```python
from build123d import *

# Parameters (mm, degrees)
SKETCH493_R     = 0.875
PAD402_DEPTH    = 1
POCKET036_DEPTH = 1.3
PAD_DEPTH       = 0.9
POCKET_DEPTH    = 2.5
CHAMFER_SIZE    = 0.1


with BuildPart() as part:
    # Sketch493 → Pad402 (new body, symmetric)
    with BuildSketch(Plane(origin=(50, -50, 0.5), x_dir=(1, 0, 0), z_dir=(0, 0, 1))):
        with BuildLine():
            Line((-53.3, 47.9), (-53.3, 46.1))
            Line((-53.3, 46.1), (-52.917836, 46.1))
            ThreePointArc((-52.73607, 46.021642), (-52.818868, 46.079576), (-52.917836, 46.1))
            ThreePointArc((-52.73607, 46.021642), (-52.488396, 45.812963), (-52.2, 45.665599))
            Line((-52.2, 45.665599), (-52.2, 45.141069))
            ThreePointArc((-52.2, 45.141069), (-50.38471, 45.594427), (-49.812013, 47.375671))
            ThreePointArc((-47.375671, 49.812013), (-49.245018, 49.245018), (-49.812013, 47.375671))
            ThreePointArc((-47.375671, 49.812013), (-45.594427, 50.38471), (-45.141069, 52.2))
            Line((-45.665599, 52.2), (-45.141069, 52.2))
            ThreePointArc((-45.665599, 52.2), (-45.812963, 52.488396), (-46.021642, 52.73607))
            ThreePointArc((-46.1, 52.917836), (-46.079576, 52.818868), (-46.021642, 52.73607))
            Line((-46.1, 53.3), (-46.1, 52.917836))
            Line((-47.9, 53.3), (-46.1, 53.3))
            Line((-47.9, 53.3), (-47.9, 52.917836))
            ThreePointArc((-47.978358, 52.73607), (-47.920424, 52.818868), (-47.9, 52.917836))
            ThreePointArc((-47.978358, 52.73607), (-48.187037, 52.488396), (-48.334401, 52.2))
            Line((-48.334401, 52.2), (-51.75, 52.2))
            ThreePointArc((-51.75, 52.2), (-52.068198, 52.068198), (-52.2, 51.75))
            Line((-52.2, 51.75), (-52.2, 48.334401))
            ThreePointArc((-52.2, 48.334401), (-52.488396, 48.187037), (-52.73607, 47.978358))
            ThreePointArc((-52.917836, 47.9), (-52.818868, 47.920424), (-52.73607, 47.978358))
            Line((-52.917836, 47.9), (-53.3, 47.9))
        make_face()
        with Locations((-50, 50)):
            Circle(SKETCH493_R, mode=Mode.SUBTRACT)
    extrude(amount=PAD402_DEPTH, both=True)

    # Sketch494 → Pocket036 (cut)
    with BuildSketch(Plane(origin=(50, -50, 1.5), x_dir=(1, 0, 0), z_dir=(0, 0, 1))):
        with BuildLine():
            Line((0, 0), (-100, 0))
            Line((-100, 0), (-100, 51.8))
            ThreePointArc((-51.8, 100), (-85.882547, 85.882547), (-100, 51.8))
            Line((-51.8, 100), (0, 100))
            Line((0, 100), (0, 0))
        make_face()
    extrude(amount=-POCKET036_DEPTH, mode=Mode.SUBTRACT)

    # Sketch497 → Pad (join)
    with BuildSketch(Plane(origin=(50, -50, 0), x_dir=(1, 0, 0), z_dir=(0, 0, 1))):
        with BuildLine():
            Line((-53.3, 47.9), (-53.3, 46.1))
            Line((-53.3, 46.1), (-52.917836, 46.1))
            ThreePointArc((-52.73607, 46.021642), (-52.818868, 46.079576), (-52.917836, 46.1))
            ThreePointArc((-52.73607, 46.021642), (-50.275, 47), (-52.73607, 47.978358))
            ThreePointArc((-52.917836, 47.9), (-52.818868, 47.920424), (-52.73607, 47.978358))
            Line((-52.917836, 47.9), (-53.3, 47.9))
        make_face()
        with BuildLine():
            Line((-46.1, 53.3), (-46.1, 52.917836))
            ThreePointArc((-46.1, 52.917836), (-46.079576, 52.818868), (-46.021642, 52.73607))
            ThreePointArc((-47.978358, 52.73607), (-47, 50.275), (-46.021642, 52.73607))
            ThreePointArc((-47.978358, 52.73607), (-47.920424, 52.818868), (-47.9, 52.917836))
            Line((-47.9, 53.3), (-47.9, 52.917836))
            Line((-47.9, 53.3), (-46.1, 53.3))
        make_face()
    extrude(amount=-PAD_DEPTH)

    # Sketch → Pocket (cut, symmetric)
    with BuildSketch(Plane(origin=(50, -50, 0), x_dir=(1, 0, 0), z_dir=(0, 0, 1))):
        Polygon((-52.2, 44.2), (-44.2, 52.2), (-42, 52.2), (-52.2, 42), align=None)
    extrude(amount=POCKET_DEPTH, both=True, mode=Mode.SUBTRACT)

    # Chamfer
    chamfer_edges = [part.edges().sort_by_distance(p)[0] for p in [
        (4.15, 0.55, 0.2),
        (4.878226, 1.278226, -0.15),
        (4.15, 0.55, -0.5),
        (3.421774, -0.178226, -0.15),
        (-0.55, -4.15, 0.2),
        (0.178226, -3.421774, -0.15),
        (-0.55, -4.15, -0.5),
        (-1.278226, -4.878226, -0.15),
    ]]
    chamfer(chamfer_edges, length=CHAMFER_SIZE)


solid = part.part
```
Model file for the job. Use its own axes, mm. A direction names the side the tool comes from. Give positions to 0.01 mm unless a question says otherwise; leave off trailing zeros. Order: outer loops, then holes, each group sorted by start corner. A loop starts at its lowest first (then second) coordinate and runs counter-clockwise, first axis right, second up.
1) Saw through at C-C, the plane y = -0.75. Write the cut outline in (x, z), then the cut area to 3 significant figures.
2) Saw through at D-D, the plane x = 3. Write the cut outline in (y, z) (3 decimals), then the cut area to 3 significant figures.
3) Saw through at B-B, the plane x = 0.5. Write the cut outline in (y, z), then the cut area to 3 significant figures.
4) 3-axis set-ups, long thin cutter, end or side, ignore diameter. For faces 1 (the flat face through (-1, 1, -0.5)), 2 (the cylindrical face through (0.808, -0.335, -0.155)): which of +Z, -Z, +X, -X, +Y, -Y reach the whole face in a straight line?
5) Wall check: probe 1 along Z at (x, y) = (1, 0); probe 2 along X at (y, z) = (0, -0.05) (3 decimals); probe 3 along Y at (x, z) = (0, 0) (3 decimals). Give the ranges that are in metal, low to high.
6) Mould opens along X. For faces 3 (the flat face through (4.1, 0.5, -0.1)), 4 (the flat face through (-2, -3, -0.9)), 5 (the cylindrical face through (0.78, -0.73, -0.15)) say: +X half, -X half, draft (parallel to the pull), parting line (faces both ways), or undercut.
Computed:
1. outline: (-2.2, -0.5) - (-0.45, -0.5) - (-0.45, 0.2) - (-2.2, 0.2) - close; (0.45, -0.5) - (0.76, -0.5) - (0.76, 0.2) - (0.45, 0.2) - close
1. area: 1.44 mm2
2. outline: (-0.225, -0.5) - (0.275, -0.5) - (0.275, -0.9) - (3.3, -0.9) - (3.3, 0.2) - (-0.225, 0.2) - close
2. area: 3.68 mm2
3. outline: (-1.06, -0.5) - (-0.72, -0.5) - (-0.72, 0.2) - (-1.06, 0.2) - close; (0.72, -0.5) - (2.2, -0.5) - (2.2, 0.2) - (0.72, 0.2) - close
3. area: 1.28 mm2
4. face 1: -Z
4. face 2: +Z, -Z
5. probe 1: z = -0.5 to 0.2
5. probe 2: x = -2.2 to -0.875, 0.875 to 3.6
5. probe 3: y = -3.6 to -0.875, 0.875 to 2.2
6. face 3: +X half
6. face 4: draft
6. face 5: undercut
